CAD build for the part. Positions are in the model's coordinates, mm. A direction names the side the tool comes from. Round coordinates to 2 decimals unless told otherwise and drop trailing zeros. Loops run counter-clockwise (first coordinate to the right, second up) from the corner with the lowest first, then second, coordinate; pieces in that order, holes last. Notation, with made-up numbers: (78.25, -16.5) - (85.25, -16.5) arc R28 ccw to (85.25, 14.5) - close; hole circle Ø9 at (-14.5, -2.75). An arc over 180 degrees is marked (long way). One line per question, with ' | ' between items.
```python
from build123d import *

# Parameters (mm, degrees)
SKETCH_1_W          = 54
SKETCH_1_H          = 25
EXTRUDE_1_DEPTH     = 5
SKETCH_2_W          = 50
SKETCH_2_H          = 22
CUT_EXTRUDE_1_DEPTH = 3
SKETCH_3_R          = 1.05
CUT_EXTRUDE_2_DEPTH = 17
SKETCH_4_W          = 15
SKETCH_4_H          = 5
CUT_EXTRUDE_3_DEPTH = 18


with BuildPart() as part:
    # 草圖1 → 填料-伸長1 (new body)
    with BuildSketch(Plane.XY):
        with Locations((10.036827119, -5.081562568)):
            Rectangle(SKETCH_1_W, SKETCH_1_H)
    extrude(amount=EXTRUDE_1_DEPTH)

    # 草圖2 → 除料-伸長1 (cut)
    with BuildSketch(Plane.XY):
        with Locations((10.036827119, -6.581562568)):
            Rectangle(SKETCH_2_W, SKETCH_2_H)
    extrude(amount=CUT_EXTRUDE_1_DEPTH, mode=Mode.SUBTRACT)

    # 草圖3 → 除料-伸長2 (cut)
    with BuildSketch(Plane.XY):
        with Locations((29.986827119, -15.931562568)):
            Circle(SKETCH_3_R)
        with Locations((-9.913172881, 2.768437432)):
            Circle(SKETCH_3_R)
    extrude(amount=CUT_EXTRUDE_2_DEPTH, mode=Mode.SUBTRACT)

    # 草圖4 → 除料-伸長3 (cut)
    with BuildSketch(Plane.XY):
        with Locations((10.036827119, -15.081562568)):
            Rectangle(SKETCH_4_W, SKETCH_4_H)
    extrude(amount=CUT_EXTRUDE_3_DEPTH, mode=Mode.SUBTRACT)


solid = part.part
```
(1) Cut at D-D, the plane z = 4.4. Write the cut outline in (x, y), then the cut area to 3 significant figures.
Results found:
outline: (-16.96, -17.58) - (2.54, -17.58) - (2.54, -12.58) - (17.54, -12.58) - (17.54, -17.58) - (37.04, -17.58) - (37.04, 7.42) - (-16.96, 7.42) - close; hole circle Ø2.1 at (-9.91, 2.77); hole circle Ø2.1 at (29.99, -15.93) | area: 1,270 mm²
(2) Cut at A-A, the plane z = 1.15. Write the cut outline in (x, y), then the cut area to 3 significant figures.
Results found:
outline: (-16.96, -17.58) - (-14.96, -17.58) - (-14.96, 4.42) - (35.04, 4.42) - (35.04, -17.58) - (37.04, -17.58) - (37.04, 7.42) - (-16.96, 7.42) - close | area: 250 mm²
(3) Drop flat-ended pins along their axis: P1, Ø2.5, axis at x = -9.91, y = 2.77, coming from the -Z side; P2, Ø1.5, axis at x = -0.5, z = 2, coming from the -Y side; P3, Ø0.6, axis at x = 9, z = 4, coming from the -Y side. Give the stop position or say it passes through.
Results found:
P1: stops at z = 3 | P2: stops at y = 4.42 | P3: stops at y = -12.58
(4) Two-plate mould, pull along Y, no slides. Class faces 4 (the face through (10, 5, 0)), 5 (the face through (10, 7.418, 2)), 6 (the face through (10, 4.418, 1)), 7 (the face through (-10.962, 2.815, 3.986)): released by +Y, released by -Y, zero draft, split by the parting line, or undercut.
Results found:
face 4: zero draft | face 5: released by +Y | face 6: released by -Y | face 7: undercut
(5) Cut at B-B, the plane x = 15. Write the cut outline in (y, z).
Results found:
outline: (-12.58, 3) - (4.42, 3) - (4.42, 0) - (7.42, 0) - (7.42, 5) - (-12.58, 5) - close
(6) Probe L1, parallel to X at y = -5, z = 0.2; L2, parallel to X at y = -14, z = 3.55; L3, parallel to Z at x = -8, y = -10. List the from-to ranges inside material, lowest first.
Results found:
L1: x = -16.96 to -14.96, 35.04 to 37.04 | L2: x = -16.96 to 2.54, 17.54 to 37.04 | L3: z = 3 to 5
(7) Cut at C-C, the plane y = 1. Write the cut outline in (x, z).
Results found:
outline: (-16.96, 0) - (-14.96, 0) - (-14.96, 3) - (35.04, 3) - (35.04, 0) - (37.04, 0) - (37.04, 5) - (-16.96, 5) - close
(8) Tool access for faces 1 (the face through (-16.963, -5, 2)), 2 (the face through (10, -6, 3)), 3 (the face through (10, -12.582, 4)): list every direction of +Z, -Z, +X, -X, +Y, -Y with a clear straight run to the whole face (end or side of a thin tool).
Results found:
face 1: +Z, -Z, -X, +Y, -Y | face 2: -Z, -Y | face 3: +Z, -Z, -Y
